```python
from build123d import *

# Parameters (mm, degrees)
F0_W     = 20
F0_H     = 560
F1_DEPTH = 500
F2_W     = 1350
F2_H     = 70
F3_DEPTH = 20
F4_W     = 1350
F4_H     = 600
F5_DEPTH = 20
F6_R     = 25
F7_DEPTH = 55
F9_DEPTH = 50


with BuildPart() as f1:
    # F0 (on Top) → F1 (new body)
    with BuildSketch(Plane.XY):
        Polygon((-675, 280), (-655, 280), (-20, 280), (0, 280), (20, 280), (655, 280), (675, 280), (675, 300), (-675, 300), align=None)
        with Locations((10, 0)):
            Rectangle(F0_W, F0_H)
        with Locations((-10, 0)):
            Rectangle(F0_W, F0_H)
    extrude(amount=F1_DEPTH)

    # F2 (on face) → F3 (join)
    with BuildSketch(Plane.XY.offset(500)):
        with Locations((0, 265)):
            Rectangle(F2_W, F2_H)
    extrude(amount=F3_DEPTH)

    # F4 (on face) → F5 (join)
    with BuildSketch(Plane(origin=(0, 0, 0), x_dir=(1, 0, 0), z_dir=(0, 0, -1))):
        Rectangle(F4_W, F4_H)
    extrude(amount=F5_DEPTH)

    # F6 (on face) → F7 (join)
    with BuildSketch(Plane(origin=(0, 0, -20), x_dir=(1, 0, 0), z_dir=(0, 0, -1))):
        with Locations((-502.596352, 223.376156)):
            Circle(F6_R)
        with Locations((-502.596352, -223.376156)):
            Circle(F6_R)
        with Locations((502.596352, -223.376156)):
            Circle(F6_R)
        with Locations((502.596352, 223.376156)):
            Circle(F6_R)
    extrude(amount=F7_DEPTH)

    # F8 (on face) → F9 (join)
    with BuildSketch(Plane(origin=(0, 0, -20), x_dir=(1, 0, 0), z_dir=(0, 0, -1))):
        Polygon((645, 270), (-645, 270), (-645, -270), (-645, -300), (-625, -300), (-625, -250), (-625, 250), (625, 250), (625, -250), (625, -300), (645, -300), (645, -270), align=None)
    extrude(amount=F9_DEPTH)


solid = f1.part
```
Source: CAD feature listing. Evaluate the final solid. Frame: model axes, mm. A direction names the side the tool comes from. Give positions to 0.01 mm unless a question says otherwise; leave off trailing zeros. Loops run counter-clockwise (first coordinate to the right, second up) from the corner with the lowest first, then second, coordinate; pieces in that order, holes last. Notation, with made-up numbers: (26, 45.5) -> (61, 45.5) arc R23 cw to (61, 71.5) -> close; hole circle Ø6 at (27, 28). An arc over 180 degrees is marked (long way). Use a Markdown table: item, result. Add a question column.
(1) Section query D-D (z = 287). Output: boundary loops of the cut face in (x, y).
(2) Access query for faces 5 (the face through (343, 255, 500)), 6 (the face through (9, -270, -45)), 7 (the face through (-645, 11, -45)). Directions: +Z, -Z, +X, -X, +Y, -Y. A direction counts if a zero-diameter tool reaches every point of the face in a straight line with its end or side. Return the directions, or none.
(3) Pull-direction query (Y, two-part tool) for faces 1 (the face through (675, 290, 131)), 2 (the face through (526.44, -230.89, -47.11)), 3 (the face through (-478.751, -230.885, -47.115)), 4 (the face through (0, -280, 246)); classes: +Y half, -Y half, draft (parallel to the pull), parting line (faces both ways), or undercut.
(4) Section query A-A (z = -39). Output: boundary loops of the cut face in (x, y), then the cut area to 3 significant figures.
(5) Ray query, line 1 (X direction, y = 161, z = -46); line 2 (Z direction, x = -102.5, y = 21.5); line 3 (Y direction, x = 137, z = -21). Return the intervals inside material, ascending.
(6) First-contact query: pin 1 Ø12 at (x, z) = (-2.5, 127.5) entering from -Y; pin 2 Ø2 at (x, y) = (242.5, 116) entering from -Z; pin 3 Ø15 at (y, z) = (-71, -37.5) entering from +X. Flat tips, straight axial feed; report the tip coordinate or a pass-through.
(7) Section query B-B (x = 383.5). Output: boundary loops of the cut face in (y, z), then the cut area to 3 significant figures.
(8) Section query C-C (y = 106). Output: boundary loops of the cut face in (x, z), then the cut area to 3 significant figures.
Checked values:
| question | item | result |
|---|---|---|
| 1 | outline | (-675, 280) -> (-20, 280) -> (-20, -280) -> (20, -280) -> (20, 280) -> (675, 280) -> (675, 300) -> (-675, 300) -> close |
| 2 | face 5 | +X, -Y |
| 2 | face 6 | -Z, +X, -X, -Y |
| 2 | face 7 | -Z, -X, +Y, -Y |
| 3 | face 1 | draft |
| 3 | face 2 | undercut |
| 3 | face 3 | undercut |
| 3 | face 4 | -Y half |
| 4 | outline | (-645, -270) -> (645, -270) -> (645, 300) -> (625, 300) -> (625, -250) -> (-625, -250) -> (-625, 300) -> (-645, 300) -> close; circle Ø50 at (-502.6, -223.38); circle Ø50 at (-502.6, 223.38); circle Ø50 at (502.6, -223.38); circle Ø50 at (502.6, 223.38) |
| 4 | area | 55,700 mm^2 |
| 5 | line 1 | -645 to -625, 625 to 645 |
| 5 | line 2 | -20 to 0 |
| 5 | line 3 | -270 to -250 |
| 6 | pin 1 | y = -280 |
| 6 | pin 2 | z = -20 |
| 6 | pin 3 | x = 645 |
| 7 | outline | (-300, -20) -> (-270, -20) -> (-270, -70) -> (-250, -70) -> (-250, -20) -> (300, -20) -> (300, 520) -> (230, 520) -> (230, 500) -> (280, 500) -> (280, 0) -> (-300, 0) -> close |
| 7 | area | 24,400 mm^2 |
| 8 | outline | (-675, -20) -> (-645, -20) -> (-645, -70) -> (-625, -70) -> (-625, -20) -> (625, -20) -> (625, -70) -> (645, -70) -> (645, -20) -> (675, -20) -> (675, 0) -> (20, 0) -> (20, 500) -> (-20, 500) -> (-20, 0) -> (-675, 0) -> close |
| 8 | area | 49,000 mm^2 |
